The model under review builds one solid part; all positions refer to its coordinate system, in mm. Face numbers are marked on the shaded views. A direction names the side the tool comes from. Round coordinates to 2 decimals unless told otherwise and drop trailing zeros. Write each loop counter-clockwise with the first axis right and the second up, starting at its lowest first coordinate (ties: lowest second). Pieces come first, ordered by that corner, then holes. Notation, with made-up numbers: (8.25, -3.75) -> (38.25, -3.75) arc R27 cw to (38.25, 15.25) -> close; hole circle Ø11 at (73.5, 44). An arc over 180 degrees is marked (long way). Answer as a JSON object with one key per item and string values. Group by question number.
1) Insertion check: pin 1 Ø0.8 at (y, z) = (-0.5, -4) entering from -X; pin 2 Ø0.6 at (y, z) = (-1, -0.5) entering from -X; pin 3 Ø1.5 at (y, z) = (1.5, -1.5) entering from -X. Each pin has a flat end and moves straight along its axis. Give the tip position at first contact, or say it passes through.
2) Machinability: for the marked faces 5 and 6, which of the approach directions +Z, -Z, +X, -X, +Y, -Y give a long, thin tool a straight path to every point of the face, cutting with its end or side? Answer none if there is none.
3) We need section B-B, the plane y = 0. Write out the cut boundary in (x, z), then the cut area to 3 significant figures.
4) We need section C-C, the plane y = -2.2. Write out the cut boundary in (x, z).
5) Mouldability with a two-part tool opening along Z and no side actions: class the marked faces 1, 2, 3 and 4 as pulls with the +Z half, pulls with the -Z half, needs draft (parallel to the pull), parting line crosses it, or undercut.
6) We need section D-D, the plane z = -0.5. Write out the cut boundary in (x, y).
7) We need section A-A, the plane x = -1.75. Write out the cut boundary in (y, z), then the cut area to 3 significant figures.
8) To check wall thickness, follow probe 1 along Y at (x, z) = (-1, 1.6); probe 2 along Z at (x, y) = (-2, -1.25); probe 3 along Z at (x, y) = (-2.25, 1.4). State the ranges of each line that lie inside material, in increasing order. Write a range as [from, to].
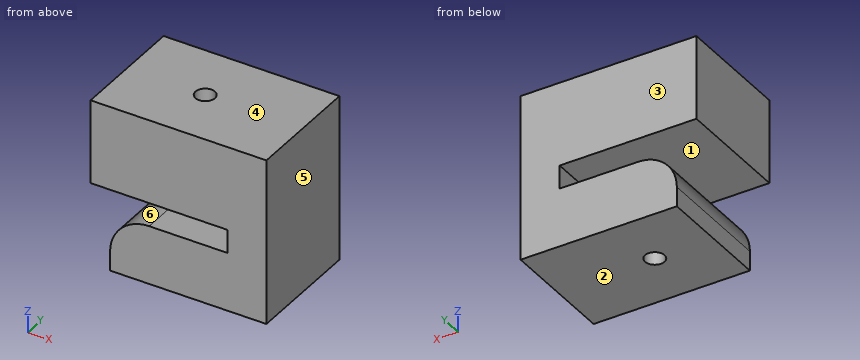
from build123d import *

# Parameters (mm, degrees)
BOSS_EXTRU_1_DEPTH      = 3
ESQUISSE3_R             = 0.5
ENL_V_MAT_EXTRU_1_DEPTH = 9.5
CONG_1_R                = 2


with BuildPart() as part:
    # Esquisse2 → Boss.-Extru.1 (new body, symmetric)
    with BuildSketch(Plane(origin=(0, 0, 0), x_dir=(1, 0, 0), z_dir=(0, 1, 0))):
        Polygon((-4, 1.25), (-4, 4.25), (4, 4.25), (4, -4.25), (-4, -4.25), (-5, -4.25), (-5, 0.05), (-4, 0.05), (2, 0.05), (2, 1.25), align=None)
    extrude(amount=BOSS_EXTRU_1_DEPTH, both=True)

    # Esquisse3 → Enlèv. mat.-Extru.1 (cut, through all)
    with BuildSketch(Plane(origin=(0, 0, -4.25), x_dir=(-1, 0, 0), z_dir=(0, 0, -1))):
        with Locations((1, 0)):
            Circle(ESQUISSE3_R)
    extrude(amount=-ENL_V_MAT_EXTRU_1_DEPTH, mode=Mode.SUBTRACT)

    # Congé1
    cong_1_edges = [part.edges().sort_by_distance(p)[0] for p in [
        (-4, 0, -1.25),
    ]]
    fillet(cong_1_edges, radius=CONG_1_R)


solid = part.part
Here are the results:
{
 "1": {"pin 1": "stops at x = -4", "pin 2": "stops at x = 2", "pin 3": "stops at x = -3.73"},
 "2": {"face 5": "+Z, -Z, +X, +Y, -Y", "face 6": "-X, +Y, -Y"},
 "3": {"outline": "(-5, -0.05) -> (-1.5, -0.05) -> (-1.5, 4.25) -> (-5, 4.25) -> close; (-4, -4.25) -> (-1.5, -4.25) -> (-1.5, -1.25) -> (-2, -1.25) arc R2 ccw to (-4, -3.25) -> close; (-0.5, -4.25) -> (4, -4.25) -> (4, 4.25) -> (-0.5, 4.25) -> (-0.5, -0.05) -> (2, -0.05) -> (2, -1.25) -> (-0.5, -1.25) -> close", "area": "56.9 mm^2"},
 "4": {"outline": "(-5, -0.05) -> (2, -0.05) -> (2, -1.25) -> (-2, -1.25) arc R2 ccw to (-4, -3.25) -> (-4, -4.25) -> (4, -4.25) -> (4, 4.25) -> (-5, 4.25) -> close"},
 "5": {"face 1": "undercut", "face 2": "pulls with the -Z half", "face 3": "needs draft", "face 4": "pulls with the +Z half"},
 "6": {"outline": "(2, -3) -> (4, -3) -> (4, 3) -> (2, 3) -> close"},
 "7": {"outline": "(-3, -4.25) -> (3, -4.25) -> (3, -1.25) -> (-3, -1.25) -> close; (-3, -0.05) -> (3, -0.05) -> (3, 4.25) -> (-3, 4.25) -> close", "area": "43.8 mm^2"},
 "8": {"probe 1": "y = [-3, -0.5], [0.5, 3]", "probe 2": "z = [-4.25, -1.25], [-0.05, 4.25]", "probe 3": "z = [-4.25, -1.27], [-0.05, 4.25]"}
}
